Could you check a few things on this model? Use its own coordinates, in mm. A direction names the side the tool comes from. Give positions to 0.01 mm unless a question says otherwise; leave off trailing zeros. Write each loop counter-clockwise with the first axis right and the second up, starting at its lowest first coordinate (ties: lowest second). Pieces come first, ordered by that corner, then holes. Notation, with made-up numbers: (54.25, 53.25) -> (108.25, 53.25) arc R10 cw to (108.25, 70.25) -> close; hole circle Ø11 at (48.5, -19). An arc over 180 degrees is marked (long way). One line per question, with ' | ' between items.
from build123d import *

# Parameters (mm, degrees)
SKETCH_6_R          = 10
CUT_EXTRUDE_4_DEPTH = 2
SKETCH_7_R          = 10
CUT_EXTRUDE_5_DEPTH = 2
SKETCH_8_R          = 10
CUT_EXTRUDE_6_DEPTH = 2
SKETCH_9_R          = 1.55
CUT_EXTRUDE_7_DEPTH = 15
SKETCH_11_W         = 3
SKETCH_11_H         = 3
CUT_EXTRUDE_9_DEPTH = 15


with BuildPart() as part:
    # 스케치1 → 회전42 (revolve)
    with BuildSketch(Plane.XY):
        with BuildLine():
            Line((0, 9), (0, -9))
            ThreePointArc((0, -9), (9, 0), (0, 9))
        make_face()
    revolve(axis=Axis((0, 9, 0), (0, -1, 0)))

    # 스케치6 → 컷-돌출4 (cut)
    with BuildSketch(Plane.XY.offset(9)):
        Circle(SKETCH_6_R)
    cut_extrude_4 = extrude(amount=-CUT_EXTRUDE_4_DEPTH, mode=Mode.SUBTRACT)

    # 대칭 복사4: 컷-돌출4 across plane
    add(cut_extrude_4.mirror(Plane.XY), mode=Mode.SUBTRACT)

    # 스케치7 → 컷-돌출5 (cut)
    with BuildSketch(Plane(origin=(0, 9, 0), x_dir=(1, 0, 0), z_dir=(0, 1, 0))):
        Circle(SKETCH_7_R)
    cut_extrude_5 = extrude(amount=-CUT_EXTRUDE_5_DEPTH, mode=Mode.SUBTRACT)

    # 대칭 복사5: 컷-돌출5 across plane
    add(cut_extrude_5.mirror(Plane.ZX), mode=Mode.SUBTRACT)

    # 스케치8 → 컷-돌출6 (cut)
    with BuildSketch(Plane(origin=(9, 0, 0), x_dir=(0, 0, -1), z_dir=(1, 0, 0))):
        Circle(SKETCH_8_R)
    cut_extrude_6 = extrude(amount=-CUT_EXTRUDE_6_DEPTH, mode=Mode.SUBTRACT)

    # 대칭 복사6: 컷-돌출6 across plane
    add(cut_extrude_6.mirror(Plane(origin=(0, 0, 0), x_dir=(0, 0, 1), z_dir=(1, 0, 0))), mode=Mode.SUBTRACT)

    # 스케치9 → 컷-돌출7 (cut, through all)
    with BuildSketch(Plane.XY.offset(7)):
        Circle(SKETCH_9_R)
    extrude(amount=-CUT_EXTRUDE_7_DEPTH, mode=Mode.SUBTRACT)

    # 스케치11 → 컷-돌출9 (cut, through all)
    with BuildSketch(Plane(origin=(7, 0, 0), x_dir=(0, 0, -1), z_dir=(1, 0, 0))):
        Rectangle(SKETCH_11_W, SKETCH_11_H)
    extrude(amount=-CUT_EXTRUDE_9_DEPTH, mode=Mode.SUBTRACT)


solid = part.part
Q1. If we mould it in two halves opening along Y, with no side actions, what happens to faces 3 (the flat face through (4, 0, 1.5)), 4 (the flat face through (-7, 0, -2)), 5 (the flat face through (0, 7, 0))? For each: +Y half, -Y half, draft (parallel to the pull), parting line (faces both ways), or undercut.
Answer below:
face 3: undercut | face 4: draft | face 5: +Y half
Q2. Imagine slicing it at C-C on x = 0. Please give me the cut outline in (y, z).
Answer below:
outline: (-7, -5.66) arc R9 ccw to (-5.66, -7) -> (-1.55, -7) -> (-1.55, 7) -> (-5.66, 7) arc R9 ccw to (-7, 5.66) -> close; (1.55, -7) -> (5.66, -7) arc R9 ccw to (7, -5.66) -> (7, 5.66) arc R9 ccw to (5.66, 7) -> (1.55, 7) -> close
Q3. Imagine slicing it at B-B on x = 4. Please give me the cut outline in (y, z).
Answer below:
outline: (-7, -4) arc R8.06 ccw to (-4, -7) -> (4, -7) arc R8.06 ccw to (7, -4) -> (7, 4) arc R8.06 ccw to (4, 7) -> (-4, 7) arc R8.06 ccw to (-7, 4) -> close; hole (-1.5, -1.5) -> (1.5, -1.5) -> (1.5, 1.5) -> (-1.5, 1.5) -> close
Q4. Imagine slicing it at D-D on z = 4.25. Please give me the cut outline in (x, y).
Answer below:
outline: (-7, -3.73) arc R7.93 ccw to (-3.73, -7) -> (3.73, -7) arc R7.93 ccw to (7, -3.73) -> (7, 3.73) arc R7.93 ccw to (3.73, 7) -> (-3.73, 7) arc R7.93 ccw to (-7, 3.73) -> close; hole circle Ø3.1 at (0, 0)
Q5. On a 3-axis mill with a long thin cutter (end or side, diameter ignored), from which of +Z, -Z, +X, -X, +Y, -Y can I reach the whole of each face in a straight line? I mean faces 1 (the flat face through (-4, 0, -1.5)), 2 (the flat face through (-1.3, -1.2, -7)). Say none if no direction works.
Answer below:
face 1: +X, -X | face 2: -Z, +X, -X, +Y, -Y
Q6. Imagine slicing it at A-A on y = 0. Please give me the cut outline in (x, z).
Answer below:
outline: (-7, -5.66) arc R9 ccw to (-5.66, -7) -> (-1.55, -7) -> (-1.55, -1.5) -> (-7, -1.5) -> close; (-7, 1.5) -> (-1.55, 1.5) -> (-1.55, 7) -> (-5.66, 7) arc R9 ccw to (-7, 5.66) -> close; (1.55, -7) -> (5.66, -7) arc R9 ccw to (7, -5.66) -> (7, -1.5) -> (1.55, -1.5) -> close; (1.55, 1.5) -> (7, 1.5) -> (7, 5.66) arc R9 ccw to (5.66, 7) -> (1.55, 7) -> close
Q7. If I drill on line 1 along Z through (x, y) = (-5, -0.5); line 2 along X through (y, z) = (0, 2.25), over which ranges is the centre line in solid material (lowest first)?
Answer below:
line 1: z = -7 to -1.5, 1.5 to 7 | line 2: x = -7 to -1.55, 1.55 to 7
